Read the model definition and answer for the solid it produces. Units are mm, in the model's axes. Face numbers are marked on the shaded views. A direction names the side the tool comes from. Round coordinates to 2 decimals unless told otherwise and drop trailing zeros. Loops run counter-clockwise (first coordinate to the right, second up) from the corner with the lowest first, then second, coordinate; pieces in that order, holes last. Notation, with made-up numbers: M -28.5,0.25 L 29.5,0.25 A18 ccw 29.5,16.25 Z; hole C 15.25,-22 d4. An arc over 180 degrees is marked long. Answer as CSV lines item,"result".
```python
from build123d import *

# Parameters (mm, degrees)
F1_ANGLE = 60
F3_DEPTH = 27
F4_R     = 2
F5_DEPTH = 15.4913810568
F6_W     = 10
F6_H     = 6
F7_DEPTH = 15.4913810568
F8_R     = 2.99999


# Not quite as in the source:
# - a fillet or chamfer is up to 0.001 mm smaller than in the source, because OpenCascade refuses the exact size


with BuildPart() as f1:
    # F0 (on Right) → F1 (revolve)
    with BuildSketch(Plane.YZ):
        Polygon((7, 0), (0, 0), (0, -2.5), (26, -2.5), (26, 0), (19, 0), (19, 2), (17, 0), (17, 2), (15, 0), (15, 2), (13, 0), (13, 2), (11, 0), (11, 2), (9, 0), (9, 2), align=None)
    revolve(axis=Axis((0, 13.3030909821, 4), (0, 1, 0)), revolution_arc=F1_ANGLE)

    # F2 (on face) → F3 (join)
    with BuildSketch(Plane.XZ):
        Polygon((10.9903810568, -6.9641016151), (-2, 0.5358983849), (-3.25, -1.6291651246), (9.7403810568, -9.1291651246), align=None)
        Polygon((-3.25, -1.6291651246), (-2, 0.5358983849), (-14.9903810568, 8.0358983849), (-16.2403810568, 5.8708348754), align=None)
    extrude(amount=-F3_DEPTH)

    # F4 (on face) → F5 (cut, through all)
    with BuildSketch(Plane(origin=(-1.5179491924, 0, -2.6291651246), x_dir=(0.8660254038, 0, -0.5), z_dir=(-0.5, 0, -0.8660254038))):
        with Locations((-13, -3)):
            Circle(F4_R)
        with Locations((9, -3)):
            Circle(F4_R)
        with Locations((-13, -13)):
            Circle(F4_R)
        with Locations((9, -13)):
            Circle(F4_R)
        with Locations((-13, -23)):
            Circle(F4_R)
        with Locations((9, -23)):
            Circle(F4_R)
    extrude(amount=-F5_DEPTH, mode=Mode.SUBTRACT)

    # F6 (on face) → F7 (cut, through all)
    with BuildSketch(Plane(origin=(-1.5179491924, 0, -2.6291651246), x_dir=(0.8660254038, 0, -0.5), z_dir=(-0.5, 0, -0.8660254038))):
        with Locations((-2, -24)):
            Rectangle(F6_W, F6_H)
    extrude(amount=-F7_DEPTH, mode=Mode.SUBTRACT)

    # F8 (radius 3 in the source; OpenCascade refuses exactly that, so slightly less here)
    f8_edges = [f1.edges().sort_by_distance(p)[0] for p in [
        (1.705127, 21, -3.046633),
        (1.705127, 27, -3.046633),
        (-6.955127, 27, 1.953367),
        (-6.955127, 21, 1.953367),
        (-15.615381, 27, 6.953367),
        (10.365381, 27, -8.046633),
    ]]
    fillet(f8_edges, radius=F8_R)


solid = f1.part
```
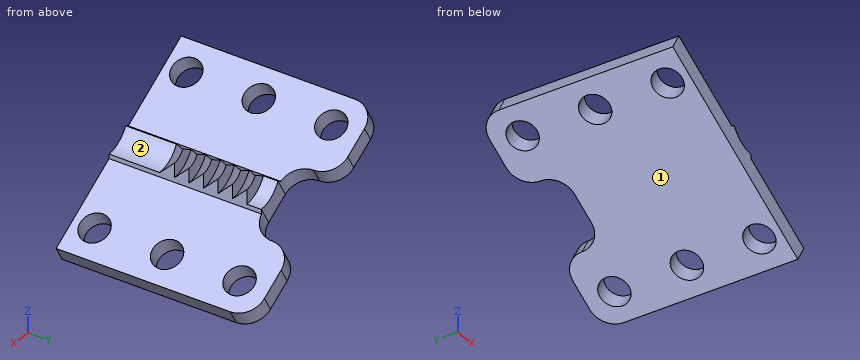
1) Straight lines are drawn through the part: line 1 (Y direction, x = -1.5, z = 1.75); line 2 (Y direction, x = 5, z = -5.75); line 3 (Y direction, x = -1.75, z = -0.5). For each, find the intervals that lie inside material, in ascending order.
Evaluation:
line 1,"y = 8.3 to 9, 10.3 to 11, 12.3 to 13, 14.3 to 15, 16.3 to 17, 18.3 to 19"
line 2,"y = 0 to 2.12, 3.88 to 12.12, 13.88 to 22.12, 23.88 to 27"
line 3,"y = 0 to 21"
2) Find section B-B, the plane x = -13. Count the separate pieces of the cut face and the enclosed holes in it, then the cut area to 3 significant figures.
Evaluation:
separate pieces,"4"
enclosed holes,"0"
area,"48.9 mm^2"
3) A tool of negligible diameter and unlimited length cuts with its end or side. For the marked faces 1 and 2, from which of +Z, -Z, +X, -X, +Y, -Y can it reach the whole face along a straight path? Write none if from no direction.
Evaluation:
face 1,"-Z, -X, +Y, -Y"
face 2,"+Z, +X, -Y"
4) Find section A-A, the plane y = 7.5. Give the vertices of the cut face in (x, z), then the cut area to 3 significant figures.
Evaluation:
outline,"M -16.24,5.87 L 9.74,-9.13 L 10.99,-6.96 L 0,-0.62 L 0,0.5 A3.5 cw -3.03,2.25 L -4,1.69 L -14.99,8.04 Z"
area,"77.8 mm^2"
5) Find section C-C, the plane y = 17.75. Give the vertices of the cut face in (x, z) (3 decimals), then the cut area to 3 significant figures.
Evaluation:
outline,"M -16.24,5.871 L 9.74,-9.129 L 10.99,-6.964 L 0,-0.619 L 0,0.75 A3.25 cw -2.815,2.375 L -4,1.691 L -14.99,8.036 Z"
area,"78.7 mm^2"
6) Each of these flat-tipped pins is pushed along its axis until it touches: P1, Ø2, axis at x = 6.5, y = 10.5, coming from the -Z side; P2, Ø0.9, axis at x = -1, z = 1, coming from the +Y side; P3, Ø4, axis at x = 6, y = 24, coming from the +Z side. Where does it stop, or does it pass through?
Evaluation:
P1,"stops at z = -7.84"
P2,"stops at y = 19"
P3,"stops at z = -2.93"
